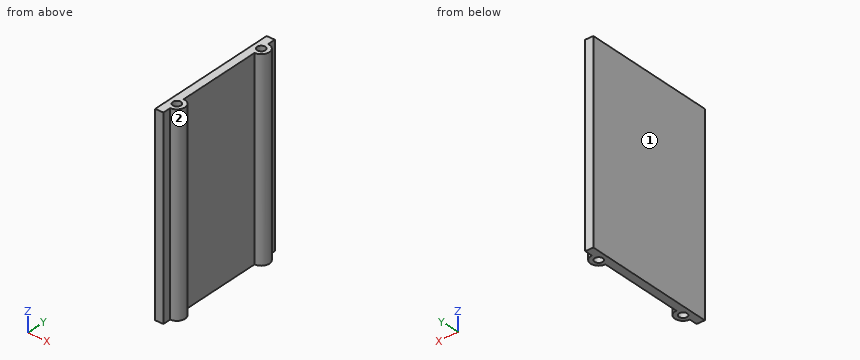
```python
from build123d import *

# Parameters (mm, degrees)
SKETCH_1_R      = 2.5
EXTRUDE_1_DEPTH = 119


with BuildPart() as part:
    # 草图1 → 凸台-拉伸1 (new body)
    with BuildSketch(Plane.XY):
        with BuildLine():
            Line((-166.5, 31.210634294), (-166.5, -31.210634294))
            Line((-166.5, -31.210634294), (-166.5, -36.210634294))
            Line((-166.5, -36.210634294), (-166.5, -41.210634294))
            Line((-166.5, -41.210634294), (-161.5, -41.210634294))
            Line((-161.5, -41.210634294), (-161.5, -36.210634294))
            ThreePointArc((-161.5, -36.210634294), (-156.5, -31.210634294), (-161.5, -26.210634294))
            Line((-161.5, -26.210634294), (-161.5, 26.210634294))
            ThreePointArc((-161.5, 26.210634294), (-156.5, 31.210634294), (-161.5, 36.210634294))
            Line((-161.5, 36.210634294), (-161.5, 41.210634294))
            Line((-161.5, 41.210634294), (-166.5, 41.210634294))
            Line((-166.5, 41.210634294), (-166.5, 36.210634294))
            Line((-166.5, 36.210634294), (-166.5, 31.210634294))
        make_face()
        with Locations((-161.5, 31.210634294)):
            Circle(SKETCH_1_R, mode=Mode.SUBTRACT)
        with Locations((-161.5, -31.210634294)):
            Circle(SKETCH_1_R, mode=Mode.SUBTRACT)
    extrude(amount=EXTRUDE_1_DEPTH)


solid = part.part
```
Read the model definition and answer for the solid it produces. Units are mm, in the model's axes. Face numbers are marked on the shaded views. Give positions to 0.01 mm unless a question says otherwise; leave off trailing zeros. Write each loop counter-clockwise with the first axis right and the second up, starting at its lowest first coordinate (ties: lowest second). Pieces come first, ordered by that corner, then holes. Notation, with made-up numbers: M -32.75,-0.75 L -4.75,-0.75 A14 ccw -4.75,22.25 Z; hole C 70.25,80.5 d6. An arc over 180 degrees is marked long. Put each result on its own line as item: value. Start each with the question number.
1. For a pull along Y with two mould halves and no side action, classify the marked faces 1 and 2 as released by +Y, released by -Y, zero draft, split by the parting line, or undercut.
2. Consider line 1 along Y through (x, z) = (-163.75, 83.5); line 2 along X through (y, z) = (-23, 98.5); line 3 along Y through (x, z) = (-159.5, 30). Determine where each line is inside the solid, lowest interval first.
3. The part is cut by section A-A, the plane z = 39. Give the vertices of the cut face in (x, y).
4. Each of these flat-tipped pins is pushed along its axis until it touches: pin 1 Ø2 at (x, z) = (-159, 90) entering from -Y; pin 2 Ø1.5 at (x, z) = (-159, 38.5) entering from +Y; pin 3 Ø2 at (x, z) = (-158.5, 63.5) entering from +Y; pin 4 Ø4 at (x, y) = (-159.5, 32) entering from -Z. Where does it stop, or does it pass through?
5. The part is cut by section B-B, the plane y = 0. Give the vertices of the cut face in (x, z), and give its area (3 significant figures).
Final values:
1. face 1: zero draft
1. face 2: undercut
2. line 1: y = -41.21 to -32.3, -30.12 to 30.12, 32.3 to 41.21
2. line 2: x = -166.5 to -161.5
2. line 3: y = -35.79 to -32.71, -29.71 to -26.63, 26.63 to 29.71, 32.71 to 35.79
3. outline: M -166.5,-41.21 L -161.5,-41.21 L -161.5,-36.21 A5 ccw -161.5,-26.21 L -161.5,26.21 A5 ccw -161.5,36.21 L -161.5,41.21 L -166.5,41.21 Z; hole C -161.5,-31.21 d5; hole C -161.5,31.21 d5
4. pin 1: stops at y = -35.98
4. pin 2: stops at y = 35.89
4. pin 3: stops at y = 35.79
4. pin 4: stops at z = 0
5. outline: M -166.5,0 L -161.5,0 L -161.5,119 L -166.5,119 Z
5. area: 595 mm²
